Read the model definition and answer for the solid it produces. Units are mm, in the model's axes. Give positions to 0.01 mm unless a question says otherwise; leave off trailing zeros. Order: outer loops, then holes, each group sorted by start corner. A loop starts at its lowest first (then second) coordinate and runs counter-clockwise, first axis right, second up.
```python
from build123d import *

# Parameters (mm, degrees)
F0_R     = 2.75
F1_DEPTH = 25


# Not quite as in the source:
# - a feature of the source that left no trace in its solid (it failed there, or was rolled back) is left out


with BuildPart() as f1:
    # F0 (on Front) → F1 (new body)
    with BuildSketch(Plane.XZ):
        Polygon((0, 3.25), (-16.5, 2.5), (-16.5, -2.5), (0, -3.25), (16.5, -2.5), (16.5, 2.5), align=None)
        Circle(F0_R, mode=Mode.SUBTRACT)
        with BuildLine():
            Line((-16.5, -2.5), (-16.5, 2.5))
            ThreePointArc((-16.5, 2.5), (-19, 0), (-16.5, -2.5))
        make_face()
        with BuildLine():
            ThreePointArc((16.5, -2.5), (19, 0), (16.5, 2.5))
            Line((16.5, 2.5), (16.5, -2.5))
        make_face()
    extrude(amount=F1_DEPTH)


solid = f1.part
```
1) The part is cut by section D-D on x = 5.5. Determine the outline of the cut face in (y, z).
Final values:
outline: (-25, -3) - (0, -3) - (0, 3) - (-25, 3) - close
2) Consider L1, parallel to Z at x = 0, y = -8.25; L2, parallel to X at y = -19.75, z = -0.75; L3, parallel to X at y = -23.5, z = 1. Determine where each line is inside the solid, lowest interval first.
Final values:
L1: z = -3.25 to -2.75, 2.75 to 3.25
L2: x = -18.88 to -2.65, 2.65 to 18.88
L3: x = -18.79 to -2.56, 2.56 to 18.79
3) The part is cut by section C-C on x = -2. Determine the outline of the cut face in (y, z), and give its area (3 significant figures).
Final values:
outline: (-25, -3.16) - (0, -3.16) - (0, -1.89) - (-25, -1.89) - close; (-25, 1.89) - (0, 1.89) - (0, 3.16) - (-25, 3.16) - close
area: 63.6 mm2
4) The part is cut by section B-B on y = -12.75. Determine the outline of the cut face in (x, z).
Final values:
outline: (-16.5, -2.5) - (0, -3.25) - (16.5, -2.5) arc R2.5 ccw to (16.5, 2.5) - (0, 3.25) - (-16.5, 2.5) arc R2.5 ccw to start; hole circle Ø5.5 at (0, 0)
5) For a pull along X with two mould halves and no side action, classify faces 1 (the face through (0, -25, -3)), 2 (the face through (-0.596, -12.325, -2.685)), 3 (the face through (8.13, -12.32, -2.88)), 4 (the face through (-19, -12, 0)) as released by +X, released by -X, zero draft, split by the parting line, or undercut.
Final values:
face 1: zero draft
face 2: undercut
face 3: released by +X
face 4: released by -X
6) Given pin 1 (1.5 mm diameter, centred on x = 14.5, y = -20, fed in from +Z) (3 decimals); pin 2 (3 mm diameter, centred on y = -15, z = 2, fed in from -X); pin 3 (3 mm diameter, centred on x = 6, z = -1.5, fed in from +Y); pin 4 (1.5 mm diameter, centred on y = -15.5, z = 2.5, fed in from +X), each flat-ended and moving along its own axis, determine where each tip first touches the part or whether it passes through.
Final values:
pin 1: stops at z = 2.625
pin 2: stops at x = -18.95
pin 3: stops at y = 0
pin 4: stops at x = 18.29
7) The part is cut by section A-A on z = 0. Determine the outline of the cut face in (x, y).
Final values:
outline: (-19, -25) - (-2.75, -25) - (-2.75, 0) - (-19, 0) - close; (2.75, -25) - (19, -25) - (19, 0) - (2.75, 0) - close
